Part print with two shaded views. Sizes in mm from the minimum x, y, z corner. A direction names the side the tool comes from. Round coordinates to 2 decimals unless told otherwise and drop trailing zeros. Order: outer loops, then holes, each group sorted by start corner. A loop starts at its lowest first (then second) coordinate and runs counter-clockwise, first axis right, second up. Notation, with made-up numbers: M 72.5,79 L 76.5,79 A15 cw 76.5,89 Z; hole C -13,15 d10. An arc over 180 degrees is marked long. One line per question, with ' | ' between items.
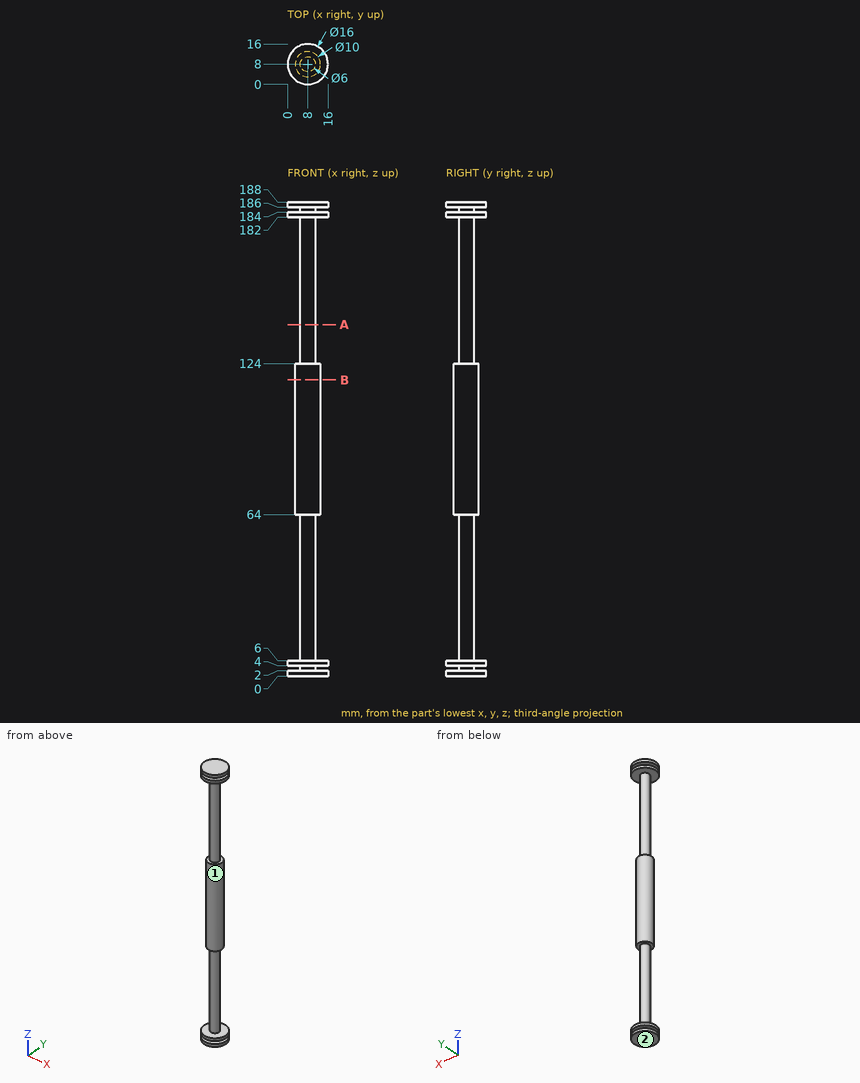
1) Probe line 1 (Z direction, x = 10.5, y = 12.5); line 2 (Z direction, x = 4.75, y = 7); line 3 (Y direction, x = 5.5, z = 54). List the from-to ranges inside material, lowest first. Write a range as [from, to].
The answers:
line 1: z = [0, 2], [4, 6], [182, 184], [186, 188] | line 2: z = [0, 2], [4, 6], [64, 124], [182, 184], [186, 188] | line 3: y = [6.34, 9.66]
2) Saw through at A-A (z = 139.5). List the corners of the cut face in (x, y), plus the area to 3 significant figures.
The answers:
outline: C 8,8 d6 | area: 28.3 mm²
3) Drop flat-ended pins along their axis: pin 1 (1.5 mm diameter, centred on y = 10.5, z = 82.5, fed in from -X); pin 2 (5 mm diameter, centred on x = 5, z = 121, fed in from -Y); pin 3 (1.5 mm diameter, centred on y = 7, z = 71, fed in from -X). Give the stop position or say it passes through.
The answers:
pin 1: stops at x = 3.32 | pin 2: stops at y = 3.03 | pin 3: stops at x = 3.01
4) Which spindle directions (+Z, -Z, +X, -X, +Y, -Y) get a long thin tool onto all of the face, cutting with end or side? Do the marked faces 1 and 2. Say none if no direction does.
The answers:
face 1: none | face 2: -Z, +X, -X, +Y, -Y
5) Saw through at B-B (z = 117.5). List the corners of the cut face in (x, y), plus the area to 3 significant figures.
The answers:
outline: C 8,8 d10 | area: 78.5 mm²
